from build123d import *

# Parameters (mm, degrees)
PAD_DEPTH       = 3
SKETCH001_R     = 1.5
POCKET_DEPTH    = 3.001
SKETCH002_R     = 5
PAD001_DEPTH    = 3
POCKET001_DEPTH = 3
SKETCH004_R     = 1.5
POCKET002_DEPTH = 3.001


with BuildPart() as part:
    # Sketch → Pad (new body)
    with BuildSketch(Plane.XY):
        with BuildLine():
            Line((48.521288, 5.237141), (39.521288, 5.237141))
            Line((39.521288, 5.237141), (39.521288, 14.237141))
            Line((39.521288, 14.237141), (-0.478712, 14.237141))
            ThreePointArc((-0.478712, 14.237141), (-5.478728, 9.23715), (-0.478728, 4.237141))
            Line((-0.478728, 4.237141), (26.564369, 4.237141))
            ThreePointArc((31.474962, 1.205189), (29.449965, 3.418084), (26.564369, 4.237141))
            ThreePointArc((31.474962, 1.205189), (34.793052, -2.420782), (39.521288, -3.762859))
            Line((39.521288, -3.762859), (48.521288, -3.762859))
            Line((48.521288, -3.762859), (48.521288, 5.237141))
        make_face()
    extrude(amount=PAD_DEPTH)

    # Sketch001 → Pocket (cut, through all)
    with BuildSketch(Plane.XY.offset(3)):
        with Locations((35.021288, 9.737141)):
            Circle(SKETCH001_R)
    extrude(amount=-POCKET_DEPTH, mode=Mode.SUBTRACT)

    # Sketch002 → Pad001 (new body)
    with BuildSketch(Plane.XY.offset(3)):
        with Locations((-0.478728, 9.237141)):
            Circle(SKETCH002_R)
    extrude(amount=PAD001_DEPTH)

    # Sketch003 → Pocket001 (cut)
    with BuildSketch(Plane.XY.offset(6)):
        Polygon((-1.853728, 11.618711), (0.896272, 11.618711), (2.271272, 9.237141), (0.896272, 6.855571), (-1.853728, 6.855571), (-3.228728, 9.237141), align=None)
    extrude(amount=-POCKET001_DEPTH, mode=Mode.SUBTRACT)

    # Sketch004 → Pocket002 (cut, through all)
    with BuildSketch(Plane.XY.offset(3)):
        with Locations((-0.478728, 9.237141)):
            Circle(SKETCH004_R)
    extrude(amount=-POCKET002_DEPTH, mode=Mode.SUBTRACT)


solid = part.part
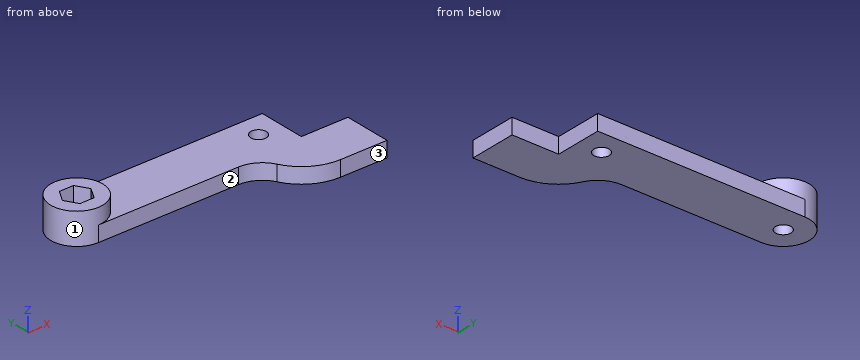
The model under review builds one solid part; all positions refer to its coordinate system, in mm. Face numbers are marked on the shaded views. A direction names the side the tool comes from. Give positions to 0.01 mm unless a question says otherwise; leave off trailing zeros. Loops run counter-clockwise (first coordinate to the right, second up) from the corner with the lowest first, then second, coordinate; pieces in that order, holes last. Notation, with made-up numbers: (14, 17) -> (35, 17) arc R26 ccw to (35, 38) -> close; hole circle Ø3 at (-35, 20.5). An arc over 180 degrees is marked (long way). Put each result on its own line as item: value. Start each with the question number.
1. We need section D-D on x = 44. State the section outline as (y, z) points, then the cut area to 3 significant figures.
2. We need section B-B on z = 4.8. State the section outline as (x, y) points, then the cut area to 3 significant figures.
3. Wall thickness on probe 1 along X at (y, z) = (9.25, 5.5); probe 2 along X at (y, z) = (9.5, 0.3); probe 3 along Z at (x, y) = (34.5, 0): over which ranges is each line inside the solid? List them lowest first.
4. Clearance check with flat-ended pins moving along their axes: P1, Ø0.9, axis at x = 12.5, z = 1.5, coming from the -Y side; P2, Ø2.5, axis at x = -0.5, y = 8.5, coming from the +Z side; P3, Ø1.5, axis at x = 44.5, z = 1, coming from the +Y side. State where each tip first meets the part, or that it passes through.
5. We need section A-A on x = 34. State the section outline as (y, z) points, then the cut area to 3 significant figures.
6. We need section C-C on z = 1.25. State the section outline as (x, y) points, then the cut area to 3 significant figures.
7. For the marked faces 1, 2 and 3, list the 3-axis set-ups (+Z, -Z, +X, -X, +Y, -Y) from which the entire face can be reached by the end or side of a thin tool; tool diameter is ignored.
Determined:
1. outline: (-3.76, 0) -> (5.24, 0) -> (5.24, 3) -> (-3.76, 3) -> close
1. area: 27.0 mm^2
2. outline: circle Ø10 at (-0.48, 9.24); hole (-3.23, 9.24) -> (-1.85, 6.86) -> (0.9, 6.86) -> (2.27, 9.24) -> (0.9, 11.62) -> (-1.85, 11.62) -> close
2. area: 58.9 mm^2
3. probe 1: -5.48 to -3.22, 2.26 to 4.52
3. probe 2: -5.47 to -1.96, 1 to 33.54, 36.5 to 39.52
3. probe 3: 0 to 3
4. P1: y = 4.24
4. P2: z = 3
4. P3: y = 5.24
5. outline: (-1.87, 0) -> (8.64, 0) -> (8.64, 3) -> (-1.87, 3) -> close; (10.84, 0) -> (14.24, 0) -> (14.24, 3) -> (10.84, 3) -> close
5. area: 41.7 mm^2
6. outline: (-0.48, 4.24) -> (26.56, 4.24) arc R5.49 cw to (31.47, 1.21) arc R9 ccw to (39.52, -3.76) -> (48.52, -3.76) -> (48.52, 5.24) -> (39.52, 5.24) -> (39.52, 14.24) -> (-0.48, 14.24) arc R5 ccw to start; hole circle Ø3 at (-0.48, 9.24); hole circle Ø3 at (35.02, 9.74)
6. area: 563 mm^2
7. face 1: +Z
7. face 2: +Z, -Z, -X, -Y
7. face 3: +Z, -Z, +X, -X, -Y
